Verification items for the finished model (mm, model axes). A direction names the side the tool comes from. Coordinates: 2 decimals unless noted, no trailing zeros. Write each loop counter-clockwise with the first axis right and the second up, starting at its lowest first coordinate (ties: lowest second). Pieces come first, ordered by that corner, then holes. Notation, with made-up numbers: M 50,30.5 L 60,30.5 A18 ccw 60,50.5 Z; hole C -19,-7.5 d1. An arc over 180 degrees is marked long. One line per item, written item: value.
```python
from build123d import *

# Parameters (mm, degrees)
BOSS_EXTRUDE1_DEPTH     = 77.5
SKETCH2_W               = 45
SKETCH2_H               = 20
BOSS_EXTRUDE2_DEPTH     = 2.5
CUT_EXTRUDE1_DEPTH      = 86.685471347
CUT_EXTRUDE1_DEPTH_BACK = 86.685471347
SKETCH3_R               = 1.5
CHAMFER3_SIZE           = 1.5
CHAMFER2_SIZE           = 1
FILLET1_R               = 1.5


with BuildPart() as part:
    # Sketch1 → Boss-Extrude1 (new body)
    with BuildSketch(Plane(origin=(0, 0, 0), x_dir=(1, 0, 0), z_dir=(0, 1, 0))):
        Polygon((12.5, -12.5), (1, -12.5), (1.866025404, -14), (-1.866025404, -14), (-1, -12.5), (-12.5, -12.5), (-12.5, -1.25), (-11, -2.116025404), (-11, 2.116025404), (-12.5, 1.25), (-12.5, 12.5), (-1.25, 12.5), (-2.116025404, 11), (2.116025404, 11), (1.25, 12.5), (12.5, 12.5), (23.75, 12.5), (22.883974596, 11), (27.116025404, 11), (26.25, 12.5), (37.5, 12.5), (37.5, 1), (39, 1.866025404), (39, -1.866025404), (37.5, -1), (37.5, -12.5), (26, -12.5), (26.866025404, -14), (23.133974596, -14), (24, -12.5), align=None)
        Polygon((15, -10), (35, -10), (35, 10), (15, 10), (10, 10), (-10, 10), (-10, -10), (10, -10), align=None, mode=Mode.SUBTRACT)
    extrude(amount=BOSS_EXTRUDE1_DEPTH)

    # Sketch2 → Boss-Extrude2 (add)
    with BuildSketch(Plane(origin=(0, 0, 0), x_dir=(1, 0, 0), z_dir=(0, 1, 0))):
        with Locations((12.5, 0)):
            Rectangle(SKETCH2_W, SKETCH2_H)
    extrude(amount=BOSS_EXTRUDE2_DEPTH)

    # Sketch3 → Cut-Extrude1 (cut, two sides: drawn at the far end of the back side and taken through both)
    with BuildSketch(Plane(origin=(0, 2.5, 0), x_dir=(1, 0, 0), z_dir=(0, 1, 0)).offset(-CUT_EXTRUDE1_DEPTH_BACK)):
        with Locations(Location((-6, 6, 0), (0, 0, 270))):
            Circle(SKETCH3_R)
        with Locations(Location((6, 6, 0), (0, 0, 270))):
            Circle(SKETCH3_R)
        with Locations(Location((6, -6, 0), (0, 0, 270))):
            Circle(SKETCH3_R)
        with Locations(Location((-6, -6, 0), (0, 0, 270))):
            Circle(SKETCH3_R)
        with Locations(Location((31, -6, 0), (0, 0, 270))):
            Circle(SKETCH3_R)
        with Locations(Location((19, -6, 0), (0, 0, 270))):
            Circle(SKETCH3_R)
        with Locations(Location((19, 6, 0), (0, 0, 270))):
            Circle(SKETCH3_R)
        with Locations(Location((31, 6, 0), (0, 0, 270))):
            Circle(SKETCH3_R)
    extrude(amount=CUT_EXTRUDE1_DEPTH + CUT_EXTRUDE1_DEPTH_BACK, mode=Mode.SUBTRACT)

    # Chamfer3
    chamfer3_edges = [part.edges().sort_by_distance(p)[0] for p in [
        (-11, 0, 0),
        (0, 0, 14),
        (25, 0, 14),
        (39, 0, 0),
        (0, 0, -11),
        (25, 0, -11),
        (-6.875, 0, -12.5),
        (-12.5, 0, -6.875),
        (-12.5, 0, 6.875),
        (-6.75, 0, 12.5),
        (12.5, 0, 12.5),
        (37.5, 0, 6.75),
        (31.75, 0, 12.5),
        (37.5, 0, -6.75),
        (31.875, 0, -12.5),
        (12.5, 0, -12.5),
    ]]
    chamfer(chamfer3_edges, length=CHAMFER3_SIZE - 0.0001)  # a hair under: the kernel refuses the full size

    # Chamfer2
    chamfer2_edges = [part.edges().sort_by_distance(p)[0] for p in [
        (12.5, 2.5, -10),
        (-10, 2.5, 0),
        (12.5, 2.5, 10),
        (35, 2.5, 0),
        (31, 2.5, 4.5),
        (-6, 2.5, 4.5),
        (6, 2.5, 4.5),
        (6, 2.5, -7.5),
        (19, 2.5, 4.5),
        (19, 2.5, -7.5),
        (31, 2.5, -7.5),
        (-6, 2.5, -7.5),
    ]]
    chamfer(chamfer2_edges, length=CHAMFER2_SIZE)

    # Fillet1
    fillet1_edges = [part.edges().sort_by_distance(p)[0] for p in [
        (35, 40.5, 10),
        (35, 40.5, -10),
        (-10, 40.5, -10),
        (-10, 40.5, 10),
    ]]
    fillet(fillet1_edges, radius=FILLET1_R)


solid = part.part
```
Item 1: Go/stop test with flat-tipped pins: P1, Ø14.5, axis at x = 10.5, z = 0.5, coming from the +Y side; P2, Ø6, axis at x = -7.5, y = 24.5, coming from the +Z side; P3, Ø3.5, axis at x = -6, z = 6, coming from the +Y side. Record where each tip stops, or that it passes through.
The answers:
P1: stops at y = 2.5
P2: stops at z = 12.5
P3: stops at y = 1.75
Item 2: Scan lines: line 1 (X direction, y = 23, z = 3.5); line 2 (X direction, y = 0.6, z = -6); line 3 (Z direction, x = 27.5, y = 45.5). Record each from-to range of solid material in increasing order.
The answers:
line 1: x = -12.5 to -10, 35 to 37.5
line 2: x = -11.6 to -7.5, -4.5 to 4.5, 7.5 to 17.5, 20.5 to 29.5, 32.5 to 36.6
line 3: z = -12.5 to -10, 10 to 12.5
Item 3: Cross-section at B-B, the plane z = 6. Give the number of separate pieces and of enclosed holes in the cut face, and give its area (3 significant figures).
The answers:
separate pieces: 5
enclosed holes: 0
area: 465 mm²
Item 4: Access from +Z, -Z, +X, -X, +Y, -Y to the whole of each face (thin tool, end or side, straight path). Record for faces 4 (the face through (-9.55, 40.8, -9.57)), 5 (the face through (-12, 1, 7)), 6 (the face through (0, 39, -11)), 7 (the face through (39, 39, 0)), 8 (the face through (-10.3, 0.8, 0)).
The answers:
face 4: +Y
face 5: +Z, -Z, -X, -Y
face 6: +Y, -Y
face 7: +Z, -Z, +X, +Y, -Y
face 8: -Y
Item 5: Draft check along X on faces 1 (the face through (38.3, 0.8, 0)), 2 (the face through (-7, 39, 12.5)), 3 (the face through (-1.719, 38.207, -11.688)). Enter one of: released by +X, released by -X, zero draft, split by the parting line, or undercut.
The answers:
face 1: released by +X
face 2: zero draft
face 3: undercut
Item 6: Cross-section at A-A, the plane x = 31. Enter the section's corners in (y, z), and give its area (3 significant figures).
The answers:
outline: M 0,-11 L 1.5,-12.5 L 77.5,-12.5 L 77.5,-10 L 3.5,-10 L 2.5,-9 L 2.5,-8.5 L 1.5,-7.5 L 0,-7.5 Z; M 0,-4.5 L 1.5,-4.5 L 2.5,-3.5 L 2.5,3.5 L 1.5,4.5 L 0,4.5 Z; M 0,7.5 L 1.5,7.5 L 2.5,8.5 L 2.5,9 L 3.5,10 L 77.5,10 L 77.5,12.5 L 1.5,12.5 L 0,11 Z
area: 419 mm²
